The listing builds one solid part. Answer for the finished solid, in the listing's coordinates (mm). Coordinates: 2 decimals unless noted, no trailing zeros. Order: outer loops, then holes, each group sorted by start corner. A loop starts at its lowest first (then second) coordinate and runs counter-clockwise, first axis right, second up. Notation, with made-up numbers: (41.25, 0.25) -> (76.25, 0.25) arc R30 ccw to (76.25, 37.25) -> close; hole circle Ø1 at (7, -32.5). An arc over 180 degrees is marked (long way). Answer in a Markdown table with one row per item.
```python
from build123d import *

# Parameters (mm, degrees)
SKETCH1_R           = 80
BOSS_EXTRUDE1_DEPTH = 5
FILLET1_R           = 2
SKETCH2_R           = 5
CUT_EXTRUDE1_DEPTH  = 5
CUT_EXTRUDE2_DEPTH  = 6


with BuildPart() as part:
    # Sketch1 → Boss-Extrude1 (new body)
    with BuildSketch(Plane(origin=(0, 0, 0), x_dir=(1, 0, 0), z_dir=(0, 1, 0))):
        Circle(SKETCH1_R)
    extrude(amount=BOSS_EXTRUDE1_DEPTH)

    # Fillet1
    fillet1_edges = [part.edges().sort_by_distance(p)[0] for p in [
        (-80, 0, 0),
        (-80, 5, 0),
    ]]
    fillet(fillet1_edges, radius=FILLET1_R)

    # Sketch2 → Cut-Extrude1 (cut)
    with BuildSketch(Plane.XZ):
        Circle(SKETCH2_R)
    extrude(amount=-CUT_EXTRUDE1_DEPTH, mode=Mode.SUBTRACT)

    # Sketch3 → Cut-Extrude2 (cut, through all)
    with BuildSketch(Plane(origin=(0, 5, 0), x_dir=(1, 0, 0), z_dir=(0, 1, 0))):
        with BuildLine():
            Line((-27, 13.5), (-27, 15))
            Line((-27, 15), (-25.5, 15))
            ThreePointArc((-25.5, 15), (-28.060660172, 16.060660172), (-27, 13.5))
        make_face()
        with BuildLine():
            Line((-25.5, 15), (-27, 15))
            Line((-27, 15), (-27, 13.5))
            ThreePointArc((-27, 13.5), (-25.939339828, 13.939339828), (-25.5, 15))
        make_face()
        with BuildLine():
            ThreePointArc((-25.5, -15), (-25.939339828, -13.939339828), (-27, -13.5))
            Line((-27, -13.5), (-27, -15))
            Line((-27, -15), (-25.5, -15))
        make_face()
        with BuildLine():
            Line((-27, -15), (-27, -13.5))
            ThreePointArc((-27, -13.5), (-28.060660172, -16.060660172), (-25.5, -15))
            Line((-25.5, -15), (-27, -15))
        make_face()
        with BuildLine():
            ThreePointArc((28.5, -15), (28.060660172, -13.939339828), (27, -13.5))
            Line((27, -13.5), (27, -15))
            Line((27, -15), (25.5, -15))
            ThreePointArc((25.5, -15), (27, -16.5), (28.5, -15))
        make_face()
        with BuildLine():
            Line((27, -15), (27, -13.5))
            ThreePointArc((27, -13.5), (25.939339828, -13.939339828), (25.5, -15))
            Line((25.5, -15), (27, -15))
        make_face()
        with BuildLine():
            ThreePointArc((28.5, 15), (27, 16.5), (25.5, 15))
            Line((25.5, 15), (27, 15))
            Line((27, 15), (27, 13.5))
            ThreePointArc((27, 13.5), (28.060660172, 13.939339828), (28.5, 15))
        make_face()
        with BuildLine():
            Line((27, 15), (25.5, 15))
            ThreePointArc((25.5, 15), (25.939339828, 13.939339828), (27, 13.5))
            Line((27, 13.5), (27, 15))
        make_face()
    extrude(amount=-CUT_EXTRUDE2_DEPTH, mode=Mode.SUBTRACT)


solid = part.part
```
(1) A cutting plane is placed at A-A, the plane x = 0. Determine the outline of the cut face in (y, z), then the cut area to 3 significant figures.
Check values:
| item | result |
|---|---|
| outline | (0, -78) arc R2 ccw to (2, -80) -> (3, -80) arc R2 ccw to (5, -78) -> (5, -5) -> (0, -5) -> close; (0, 5) -> (5, 5) -> (5, 78) arc R2 ccw to (3, 80) -> (2, 80) arc R2 ccw to (0, 78) -> close |
| area | 747 mm² |
(2) A cutting plane is placed at B-B, the plane z = 0. Determine the outline of the cut face in (x, y).
Check values:
| item | result |
|---|---|
| outline | (-80, 2) arc R2 ccw to (-78, 0) -> (-5, 0) -> (-5, 5) -> (-78, 5) arc R2 ccw to (-80, 3) -> close; (5, 0) -> (78, 0) arc R2 ccw to (80, 2) -> (80, 3) arc R2 ccw to (78, 5) -> (5, 5) -> close |
(3) Flat-ended cylindrical pins translate along their axes: pin 1 (2.5 mm diameter, centred on x = -27, z = -15, fed in from +Y); pin 2 (2 mm diameter, centred on y = 3.5, z = 60, fed in from -X). Find the tip coordinate at first contact, or state that the pin passes through.
Check values:
| item | result |
|---|---|
| pin 1 | through |
| pin 2 | x = -53.97 |
(4) Find the intervals of material crossed by line 1 along Z through (x, y) = (-27, 1.95); line 2 along X through (y, z) = (1.45, -16); line 3 along X through (y, z) = (1.55, -15), in increasing order. Write a range as from..to.
Check values:
| item | result |
|---|---|
| line 1 | -75.31..-16.5, -13.5..13.5, 16.5..75.31 |
| line 2 | -78.3..-28.12, -25.88..25.88, 28.12..78.3 |
| line 3 | -78.53..-28.5, -25.5..25.5, 28.5..78.53 |
